For this review, use the dimensioned drawing (mm, ordinates from the lowest corner) and the shaded views. A direction names the side the tool comes from. Round coordinates to 2 decimals unless told otherwise and drop trailing zeros. Loops run counter-clockwise (first coordinate to the right, second up) from the corner with the lowest first, then second, coordinate; pieces in that order, holes last. Notation, with made-up numbers: (-24, 28.5) - (35, 28.5) arc R19 ccw to (35, 40.5) - close; hole circle Ø10 at (74.5, 10). An arc over 180 degrees is marked (long way). Return JSON: item names as keys, results as strings. Group by question number.
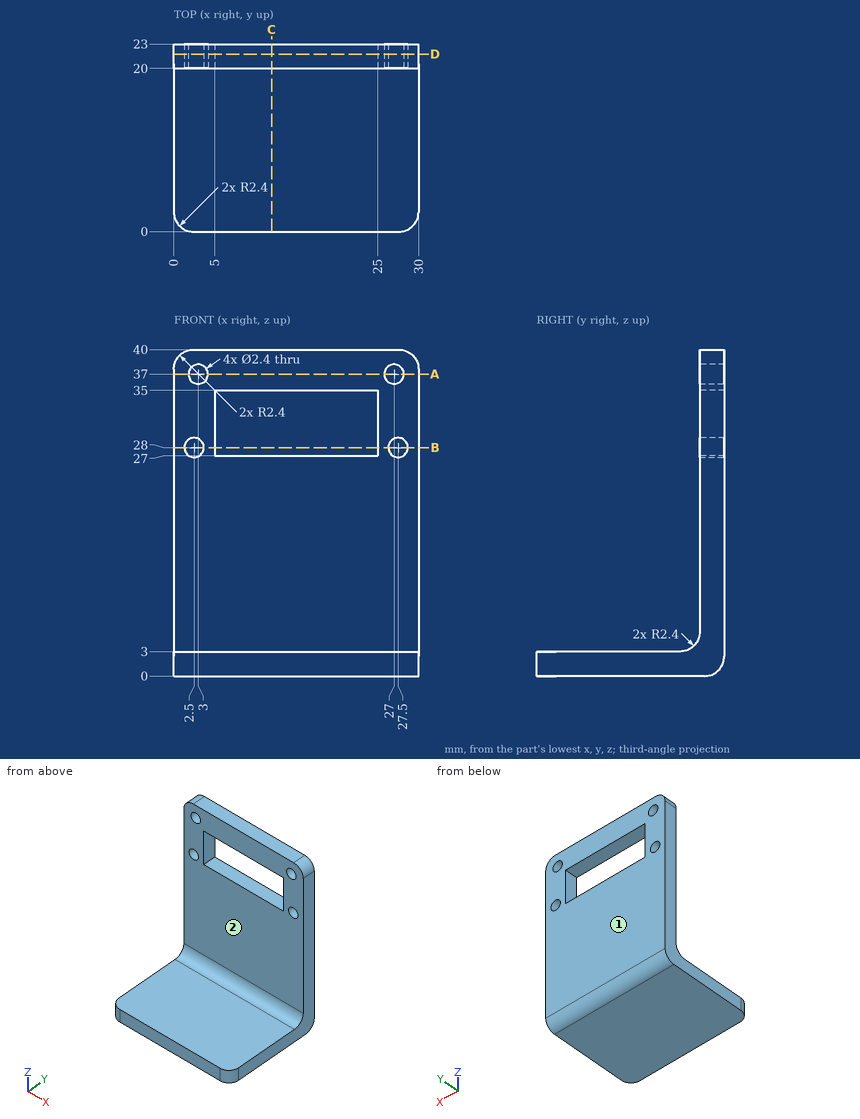
Q1. Add section A-A, the plane z = 37. State the section outline as (x, y) points, plus the area to 3 significant figures.
Q2. For line 1 (X direction, y = 20.75, z = 28); line 2 (Z direction, x = 24, y = 11.5); line 3 (Y direction, x = 16, z = 15.5), list the stretches that pass through material, from the lowest coordinate up.
Q3. Add section D-D, the plane y = 21.75. State the section outline as (x, z) points, plus the area to 3 significant figures.
Q4. Tool access review of the marked faces 1 and 2: name each direction out of +Z, -Z, +X, -X, +Y, -Y from which nothing blocks a thin tool from reaching the whole face with its end or side.
Q5. Add section B-B, the plane z = 28. State the section outline as (x, y) points, plus the area to 3 significant figures.
Q6. Insertion check: pin 1 Ø12 at (x, z) = (27, 18) entering from -Y; pin 2 Ø8 at (x, y) = (10, 3) entering from +Z. Each pin has a flat end and moves straight along its axis. Give the tip position at first contact, or say it passes through.
Q7. Add section C-C, the plane x = 12. State the section outline as (y, z) points, plus the area to 3 significant figures.
Evaluation:
{
 "1": {"outline": "(0, 20) - (1.8, 20) - (1.8, 23) - (0, 23) - close; (4.2, 20) - (25.8, 20) - (25.8, 23) - (4.2, 23) - close; (28.2, 20) - (30, 20) - (30, 23) - (28.2, 23) - close", "area": "75.6 mm²"},
 "2": {"line 1": "0 to 1.3, 3.7 to 5, 25 to 26.3, 28.7 to 30", "line 2": "0 to 3", "line 3": "20 to 23"},
 "3": {"outline": "(0, 0.29) - (30, 0.29) - (30, 37.6) arc R2.4 ccw to (27.6, 40) - (2.4, 40) arc R2.4 ccw to (0, 37.6) - close; hole circle Ø2.4 at (2.5, 28); hole circle Ø2.4 at (3, 37); hole (5, 27) - (25, 27) - (25, 35) - (5, 35) - close; hole circle Ø2.4 at (27, 37); hole circle Ø2.4 at (27.5, 28)", "area": "1,010 mm²"},
 "4": {"face 1": "+Z, -Z, +X, -X, +Y", "face 2": "+Z, +X, -X, -Y"},
 "5": {"outline": "(0, 20) - (1.3, 20) - (1.3, 23) - (0, 23) - close; (3.7, 20) - (5, 20) - (5, 23) - (3.7, 23) - close; (25, 20) - (26.3, 20) - (26.3, 23) - (25, 23) - close; (28.7, 20) - (30, 20) - (30, 23) - (28.7, 23) - close", "area": "15.6 mm²"},
 "6": {"pin 1": "y = 20", "pin 2": "z = 3"},
 "7": {"outline": "(0, 0) - (20.6, 0) arc R2.4 ccw to (23, 2.4) - (23, 27) - (20, 27) - (20, 5.4) arc R2.4 cw to (17.6, 3) - (0, 3) - close; (20, 35) - (23, 35) - (23, 40) - (20, 40) - close", "area": "156 mm²"}
}
